Design review of the part shown in the three views and the two pictorial views. Dimensions are in mm from the part's minimum x, y and z. Coordinates: 2 decimals unless noted, no trailing zeros. Write each loop counter-clockwise with the first axis right and the second up, starting at its lowest first coordinate (ties: lowest second). Pieces come first, ordered by that corner, then holes. Notation, with made-up numbers: (-21, 16.5) -> (26, 16.5) arc R14 ccw to (26, 29.5) -> close; hole circle Ø10 at (-34, 30). An arc over 180 degrees is marked (long way). Answer in a Markdown table with one row per item. Add a question column.
Item 1: Take a section at A-A, the plane y = 5. Write out the cut boundary in (x, z), and give its area (3 significant figures).
Item 2: Take a section at B-B, the plane z = 3. Write out the cut boundary in (x, y), and give its area (3 significant figures).
Item 3: To check wall thickness, follow line 1 (Y direction, x = 34, z = 2.6); line 2 (X direction, y = 7.25, z = 4.2); line 3 (X direction, y = 0.75, z = 3.9). State the ranges of each line that lie inside material, in increasing order.
Item 4: Take a section at D-D, the plane x = 14. Write out the cut boundary in (y, z).
Item 5: Take a section at C-C, the plane x = 5. Write out the cut boundary in (y, z), and give its area (3 significant figures).
Item 6: Draft analysis for pull direction Z (two halves, no side actions). For the marked faces 1, 2 and 3, state which applies: released by +Z, released by -Z, zero draft, split by the parting line, or undercut.
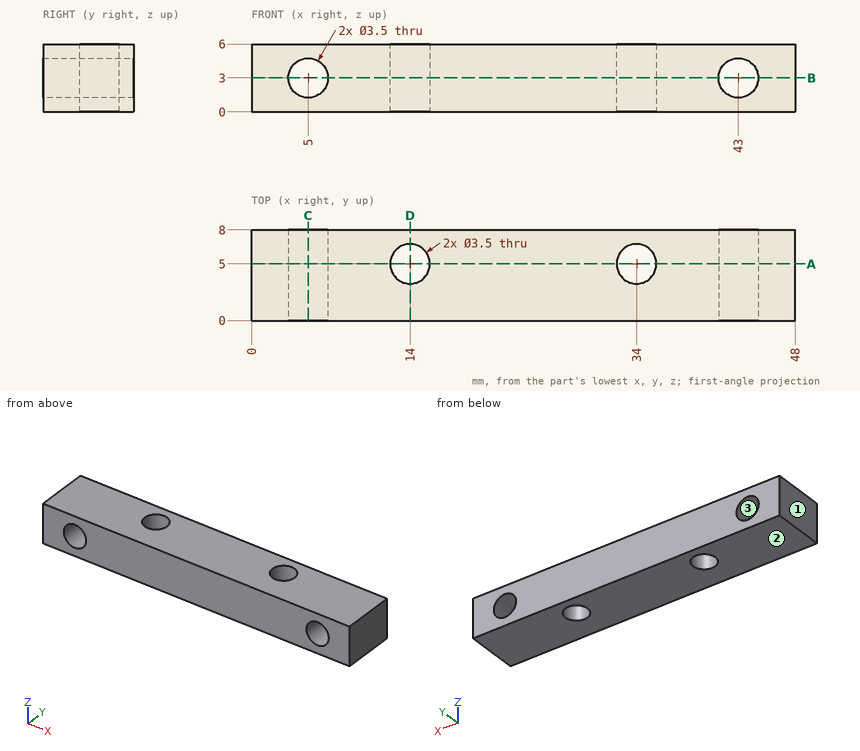
Answers:
| question | item | result |
|---|---|---|
| 1 | outline | (0, 0) -> (12.25, 0) -> (12.25, 6) -> (0, 6) -> close; (15.75, 0) -> (32.25, 0) -> (32.25, 6) -> (15.75, 6) -> close; (35.75, 0) -> (48, 0) -> (48, 6) -> (35.75, 6) -> close; hole circle Ø3.5 at (5, 3); hole circle Ø3.5 at (43, 3) |
| 1 | area | 227 mm^2 |
| 2 | outline | (0, 0) -> (3.25, 0) -> (3.25, 8) -> (0, 8) -> close; (6.75, 0) -> (41.25, 0) -> (41.25, 8) -> (6.75, 8) -> close; (44.75, 0) -> (48, 0) -> (48, 8) -> (44.75, 8) -> close; hole circle Ø3.5 at (14, 5); hole circle Ø3.5 at (34, 5) |
| 2 | area | 309 mm^2 |
| 3 | line 1 | y = 0 to 3.25, 6.75 to 8 |
| 3 | line 2 | x = 0 to 3.73, 6.27 to 41.73, 44.27 to 48 |
| 3 | line 3 | x = 0 to 3.5, 6.5 to 41.5, 44.5 to 48 |
| 4 | outline | (0, 0) -> (3.25, 0) -> (3.25, 6) -> (0, 6) -> close; (6.75, 0) -> (8, 0) -> (8, 6) -> (6.75, 6) -> close |
| 5 | outline | (0, 0) -> (8, 0) -> (8, 1.25) -> (0, 1.25) -> close; (0, 4.75) -> (8, 4.75) -> (8, 6) -> (0, 6) -> close |
| 5 | area | 20.0 mm^2 |
| 6 | face 1 | zero draft |
| 6 | face 2 | released by -Z |
| 6 | face 3 | undercut |
